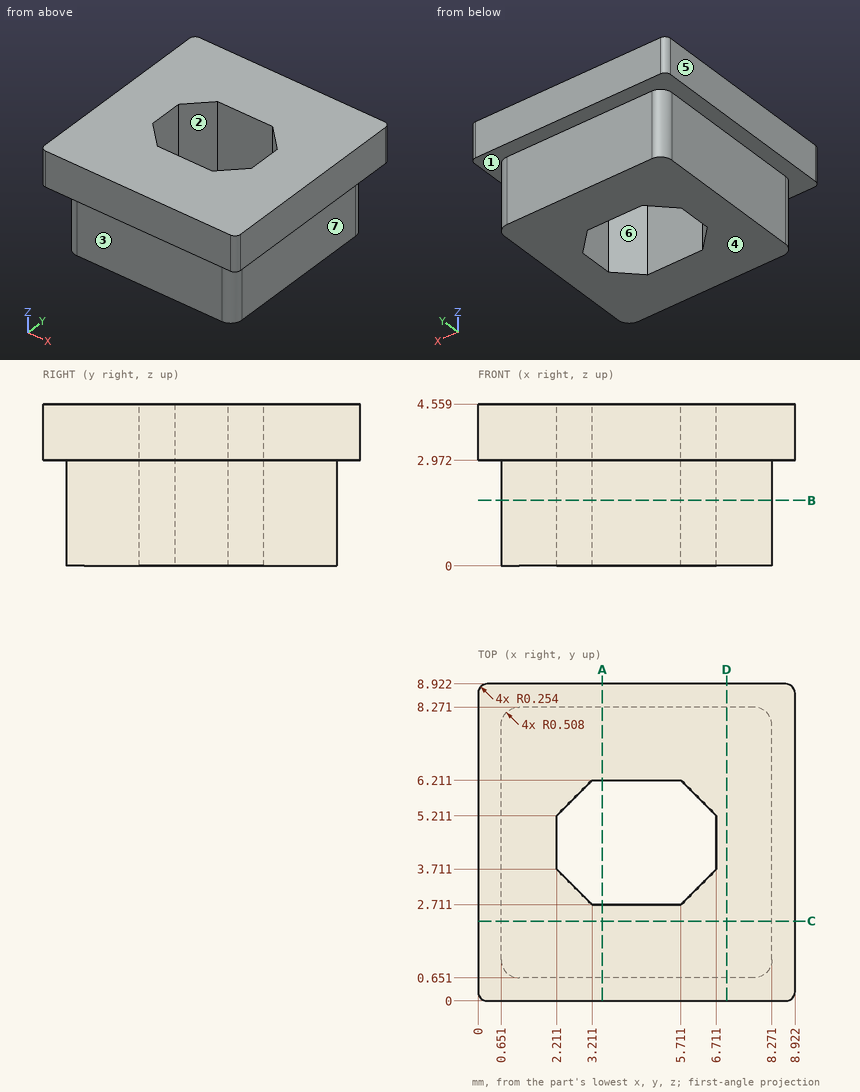
Could you check a few things on this drawing? It's one solid part, dimensions in mm from its lowest x, y, z. A direction names the side the tool comes from. Give positions to 0.01 mm unless a question says otherwise; leave off trailing zeros. Write each loop counter-clockwise with the first axis right and the second up, starting at its lowest first coordinate (ties: lowest second). Pieces come first, ordered by that corner, then holes.
(1) Imagine slicing it at B-B, the plane z = 1.85. Write out the boundary of the cut face in (x, y), and give its area (3 significant figures).
Output values:
outline: (0.65, 1.16) arc R0.51 ccw to (1.16, 0.65) - (7.76, 0.65) arc R0.51 ccw to (8.27, 1.16) - (8.27, 7.76) arc R0.51 ccw to (7.76, 8.27) - (1.16, 8.27) arc R0.51 ccw to (0.65, 7.76) - close; hole (2.21, 3.71) - (3.21, 2.71) - (5.71, 2.71) - (6.71, 3.71) - (6.71, 5.21) - (5.71, 6.21) - (3.21, 6.21) - (2.21, 5.21) - close
area: 44.1 mm2
(2) Thinking about a two-plate mould opening in X: for the marked faces 4, 5, 6 and 7, which applies, pulls with the +X half, pulls with the -X half, needs draft (parallel to the pull), parting line crosses it, or undercut?
Output values:
face 4: needs draft
face 5: pulls with the -X half
face 6: undercut
face 7: pulls with the +X half
(3) Imagine slicing it at A-A, the plane x = 3.5. Write out the boundary of the cut face in (y, z).
Output values:
outline: (0, 2.97) - (0.65, 2.97) - (0.65, 0) - (2.71, 0) - (2.71, 4.56) - (0, 4.56) - close; (6.21, 0) - (8.27, 0) - (8.27, 2.97) - (8.92, 2.97) - (8.92, 4.56) - (6.21, 4.56) - close
(4) Will these pins go through, and if not, where does the flat tip stop? pin 1 (2.5 mm diameter, centred on y = 4.5, z = 1, fed in from +X); pin 2 (0.8 mm diameter, centred on x = 4.5, z = 2, fed in from -Y); pin 3 (1.5 mm diameter, centred on x = 5.5, z = 2.5, fed in from -Y); pin 4 (2.5 mm diameter, centred on x = 5, y = 4.5, fed in from -Z).
Output values:
pin 1: stops at x = 8.27
pin 2: stops at y = 0.65
pin 3: stops at y = 0
pin 4: passes through
(5) If I drill on L1, parallel to Y at x = 5.5, z = 2.15; L2, parallel to Y at x = 2.25, z = 0.9; L3, parallel to X at y = 5.75, z = 1.25, over which ranges is the centre line in solid material (lowest first)?
Output values:
L1: y = 0.65 to 2.71, 6.21 to 8.27
L2: y = 0.65 to 3.67, 5.25 to 8.27
L3: x = 0.65 to 2.75, 6.17 to 8.27
(6) Imagine slicing it at C-C, the plane y = 2.25. Write out the boundary of the cut face in (x, z).
Output values:
outline: (0, 2.97) - (0.65, 2.97) - (0.65, 0) - (8.27, 0) - (8.27, 2.97) - (8.92, 2.97) - (8.92, 4.56) - (0, 4.56) - close
(7) On a 3-axis mill with a long thin cutter (end or side, diameter ignored), from which of +Z, -Z, +X, -X, +Y, -Y can I reach the whole of each face in a straight line? I mean the marked faces 1, 2 and 3. Say none if no direction works.
Output values:
face 1: -Z
face 2: +Z, -Z
face 3: -Z, +X, -X, -Y
